from build123d import *

# Parameters (mm, degrees)
F1_DEPTH = 30
F2_R     = 30
F3_R     = 29.99999
F4_R     = 15
F5_DEPTH = 15
F7_R     = 4
F8_DEPTH = 20


# Not quite as in the source:
# - a fillet or chamfer is up to 0.001 mm smaller than in the source, because OpenCascade refuses the exact size


with BuildPart() as f1:
    # F0 (on Front) → F1 (new body, symmetric)
    with BuildSketch(Plane.XZ):
        Polygon((-100, 0), (0, 0), (0, 35), (-20, 35), (-20, 15), (-100, 15), align=None)
    extrude(amount=F1_DEPTH, both=True)

    # F2
    f2_edges = [f1.edges().sort_by_distance(p)[0] for p in [
        (-100, -30, 7.5),
    ]]
    fillet(f2_edges, radius=F2_R)

    # F3 (radius 30 in the source; OpenCascade refuses exactly that, so slightly less here)
    f3_edges = [f1.edges().sort_by_distance(p)[0] for p in [
        (-100, 30, 7.5),
    ]]
    fillet(f3_edges, radius=F3_R)

    # F4 (on face) → F5 (cut, through all)
    with BuildSketch(Plane.XY.offset(15)):
        with Locations((-70, 0)):
            Circle(F4_R)
    extrude(amount=-F5_DEPTH, mode=Mode.SUBTRACT)

    # F6: F1 across plane


with BuildPart() as f1_1:
    add(f1.part)
    add(f1.part.mirror(Plane.XY))

    # F7 (on Right) → F8 (cut, through all)
    with BuildSketch(Plane.YZ):
        with Locations((-19.9676731229, 25.3771519661)):
            Circle(F7_R)
        with Locations((20.0323268771, 25.3771519661)):
            Circle(F7_R)
        with BuildLine():
            ThreePointArc((-23.9676731229, -24.6228480339), (-19.9676731229, -28.6228480339), (-15.9676731229, -24.6228480339))
            ThreePointArc((-15.9676731229, -24.6228480339), (-19.9676731229, -20.6228480339), (-23.9676731229, -24.6228480339))
        make_face()
        with Locations((20.0323268771, -24.6228480339)):
            Circle(F7_R)
    extrude(amount=-F8_DEPTH, mode=Mode.SUBTRACT)


solid = f1_1.part
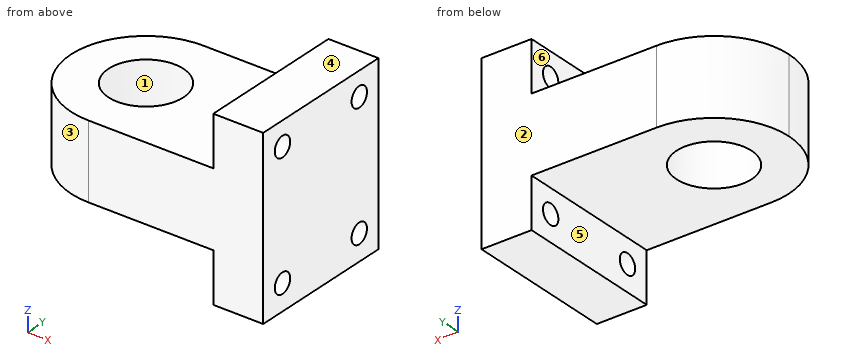
Verification items for the finished model (mm, model axes). Face numbers are marked on the shaded views. A direction names the side the tool comes from. Coordinates: 2 decimals unless noted, no trailing zeros. Write each loop counter-clockwise with the first axis right and the second up, starting at its lowest first coordinate (ties: lowest second). Pieces come first, ordered by that corner, then holes. Notation, with made-up numbers: M 5,22 L 50,22 A22 cw 50,47 Z; hole C -2,83.25 d10. An arc over 180 degrees is marked long. Use CSV: the item, a comma, the result in double quotes.
Q1. Section check B-B, the plane y = 10. Enter the section's corners in (x, z).
Computed values:
outline,"M -98.28,-15 L -81.18,-15 L -81.18,15 L -98.28,15 Z; M -58.82,-15 L -20,-15 L -20,-35 L 0,-35 L 0,35 L -20,35 L -20,15 L -58.82,15 Z"
Q2. Go/stop test with flat-tipped pins: P1, Ø6, axis at y = 8.5, z = -26, coming from the -X side; P2, Ø2, axis at y = 11, z = -6, coming from the -X side; P3, Ø8, axis at y = -10, z = -11.5, coming from the +X side; P4, Ø5, axis at y = 20.03, z = -24.62, coming from the +X side. Record where each tip stops, or that it passes through.
Computed values:
P1,"x = -20"
P2,"x = -98.28"
P3,"x = 0"
P4,"through"
Q3. Mould release check, pull along Y, two halves, no side actions. Record for the marked faces 1, 2 and 3: pulls with the +Y half, pulls with the -Y half, needs draft (parallel to the pull), parting line crosses it, or undercut.
Computed values:
face 1,"undercut"
face 2,"pulls with the +Y half"
face 3,"pulls with the -Y half"
Q4. Section check D-D, the plane z = 26.5. Enter the section's corners in (x, y), and give its area (3 significant figures).
Computed values:
outline,"M -20,-30 L 0,-30 L 0,-23.81 L -20,-23.81 Z; M -20,-16.13 L 0,-16.13 L 0,16.19 L -20,16.19 Z; M -20,23.87 L 0,23.87 L 0,30 L -20,30 Z"
area,"893 mm²"
Q5. Section check C-C, the plane x = -77. Enter the section's corners in (y, z).
Computed values:
outline,"M -29.17,-15 L -13.27,-15 L -13.27,15 L -29.17,15 Z; M 13.27,-15 L 29.17,-15 L 29.17,15 L 13.27,15 Z"
Q6. Set-up check for the marked faces 4, 5 and 6: record each of +Z, -Z, +X, -X, +Y, -Y from which the full face is reachable in a straight line by a thin tool's end or side.
Computed values:
face 4,"+Z, +X, -X, +Y, -Y"
face 5,"-Z, -X, +Y, -Y"
face 6,"+Z, -X, +Y, -Y"
Q7. Thickness scan on line 1 along Y through (x, z) = (-5, 25); line 2 along Z through (x, y) = (-8.5, -18); line 3 along X through (y, z) = (-14.5, 26.5). Record the ranges inside material, lowest first. Write a range as [from, to].
Computed values:
line 1,"[-30, -23.95], [-15.99, 16.05], [24.01, 30]"
line 2,"[-35, -28.11], [-21.14, 21.89], [28.86, 35]"
line 3,"[-20, 0]"
